The listing builds one solid part. Answer for the finished solid, in the listing's coordinates (mm). A direction names the side the tool comes from. Coordinates: 2 decimals unless noted, no trailing zeros. Write each loop counter-clockwise with the first axis right and the second up, starting at its lowest first coordinate (ties: lowest second). Pieces come first, ordered by that corner, then holes.
from build123d import *

# Parameters (mm, degrees)
F0_R     = 8
F1_DEPTH = 25
F2_R     = 2
F3_R     = 6
F4_DEPTH = 20
F5_R     = 1


with BuildPart() as f1:
    # F0 (on Top) → F1 (new body)
    with BuildSketch(Plane.XY):
        Circle(F0_R)
    extrude(amount=F1_DEPTH)

    # F2
    f2_edges = [f1.edges().sort_by_distance(p)[0] for p in [
        (-8, 0, 0),
    ]]
    fillet(f2_edges, radius=F2_R)

    # F3 (on face) → F4 (cut)
    with BuildSketch(Plane.XY.offset(25)):
        Circle(F3_R)
    extrude(amount=-F4_DEPTH, mode=Mode.SUBTRACT)

    # F5
    f5_edges = [f1.edges().sort_by_distance(p)[0] for p in [
        (-8, 0, 25),
    ]]
    fillet(f5_edges, radius=F5_R)


solid = f1.part
Q1. The part is cut by section C-C, the plane z = 18. Write down the section's boundary in (x, y), then the cut area to 3 significant figures.
Answers below:
outline: circle Ø16 at (0, 0); hole circle Ø12 at (0, 0)
area: 88.0 mm2
Q2. The part is cut by section A-A, the plane y = 0. Write down the section's boundary in (x, z), then the cut area to 3 significant figures.
Answers below:
outline: (-8, 2) arc R2 ccw to (-6, 0) - (6, 0) arc R2 ccw to (8, 2) - (8, 24) arc R1 ccw to (7, 25) - (6, 25) - (6, 5) - (-6, 5) - (-6, 25) - (-7, 25) arc R1 ccw to (-8, 24) - close
area: 158 mm2
Q3. Which of the six approach directions +Z, -Z, +X, -X, +Y, -Y give full straight-line access (tool end or side, diameter ignored) to faces 4 (the face through (0, 0, 5)), 5 (the face through (6, 2, 25))?
Answers below:
face 4: +Z
face 5: +Z, +X, -X, +Y, -Y
Q4. Find the intervals of material crossed by probe 1 along Y at (x, z) = (0, 19.75); probe 2 along X at (y, z) = (0.25, 11.5); probe 3 along Z at (x, y) = (-5, 1), in increasing order.
Answers below:
probe 1: y = -8 to -6, 6 to 8
probe 2: x = -8 to -5.99, 5.99 to 8
probe 3: z = 0 to 5
Q5. Determine the mould class of faces 1 (the face through (-1.73, -7.81, 12.85)), 2 (the face through (0, 0, 0)), 3 (the face through (-6, 0, 15)) for opening direction X: released by +X, released by -X, zero draft, split by the parting line, or undercut.
Answers below:
face 1: split by the parting line
face 2: zero draft
face 3: undercut
Q6. Given pin 1 (2 mm diameter, centred on x = -2, z = 17, fed in from +Y); pin 2 (1.5 mm diameter, centred on x = -1, z = 8, fed in from -Y); pin 3 (3 mm diameter, centred on x = 4.5, z = 17, fed in from -Y), each flat-ended and moving along its own axis, determine where each tip first touches the part or whether it passes through.
Answers below:
pin 1: stops at y = 7.94
pin 2: stops at y = -8
pin 3: stops at y = -7.42
